from build123d import *

# Parameters (mm, degrees)
SKETCH_1_W      = 53.3
SKETCH_1_H      = 68.6
SKETCH_1_R      = 1.5
EXTRUDE_1_DEPTH = 1.6
SKETCH_2_W      = 11.561255196
SKETCH_2_H      = 12.248286565
SKETCH_2_W_2    = 5.622199285
SKETCH_2_W_3    = 5.780627598
SKETCH_2_H_2    = 42.710987652
SKETCH_2_W_4    = 4.348124609
SKETCH_2_H_3    = 38.380226424
EXTRUDE_2_DEPTH = 10


with BuildPart() as part:
    # 草图1 → 凸台-拉伸1 (new body)
    with BuildSketch(Plane.XY):
        with Locations((-11.140811044, 19.148070952)):
            Rectangle(SKETCH_1_W, SKETCH_1_H)
        with Locations((-19.990811044, 50.948070952)):
            Circle(SKETCH_1_R, mode=Mode.SUBTRACT)
        with Locations((7.909188956, 50.948070952)):
            Circle(SKETCH_1_R, mode=Mode.SUBTRACT)
        with Locations((-32.490811044, 0.148070952)):
            Circle(SKETCH_1_R, mode=Mode.SUBTRACT)
        with Locations((13.009188956, -1.151929048)):
            Circle(SKETCH_1_R, mode=Mode.SUBTRACT)
    extrude(amount=EXTRUDE_1_DEPTH)

    # 草图2 → 凸台-拉伸2 (add)
    with BuildSketch(Plane.XY.offset(1.6)):
        with Locations((-26.811580019, -9.027785766)):
            Rectangle(SKETCH_2_W, SKETCH_2_H)
        with Locations((6.68110059, -9.027785766)):
            Rectangle(SKETCH_2_W_2, SKETCH_2_H)
        with Locations((-29.701893818, 25.423145352)):
            Rectangle(SKETCH_2_W_3, SKETCH_2_H_2)
        with Locations((8.855162896, 27.588525966)):
            Rectangle(SKETCH_2_W_4, SKETCH_2_H_3)
    extrude(amount=EXTRUDE_2_DEPTH)


solid = part.part
Could you check a few things on this model? Use its own coordinates, in mm. A direction names the side the tool comes from. Give positions to 0.01 mm unless a question says otherwise; leave off trailing zeros. Order: outer loops, then holes, each group sorted by start corner. A loop starts at its lowest first (then second) coordinate and runs counter-clockwise, first axis right, second up.
1. Thinking about a two-plate mould opening in X: for faces 5 (the flat face through (-21.031, -9, 7)), 6 (the flat face through (-32.592, 25, 7)), 7 (the flat face through (-27, -9, 11.6)), which applies, +X half, -X half, draft (parallel to the pull), parting line (faces both ways), or undercut?
Answers below:
face 5: undercut
face 6: -X half
face 7: draft
2. Suppose I cut it at D-D (x = -19.5). Write out the boundary of the cut face in (y, z), plus the area to 3 significant figures.
Answers below:
outline: (-15.15, 0) - (49.53, 0) - (49.53, 1.6) - (-15.15, 1.6) - close; (52.37, 0) - (53.45, 0) - (53.45, 1.6) - (52.37, 1.6) - close
area: 105 mm2
3. Suppose I cut it at C-C (y = 31.5). Write out the boundary of the cut face in (x, z).
Answers below:
outline: (-37.79, 0) - (15.51, 0) - (15.51, 1.6) - (11.03, 1.6) - (11.03, 11.6) - (6.68, 11.6) - (6.68, 1.6) - (-26.81, 1.6) - (-26.81, 11.6) - (-32.59, 11.6) - (-32.59, 1.6) - (-37.79, 1.6) - close
4. Suppose I cut it at A-A (z = 8.5). Write out the boundary of the cut face in (x, y).
Answers below:
outline: (-32.59, -15.15) - (-21.03, -15.15) - (-21.03, -2.9) - (-32.59, -2.9) - close; (-32.59, 4.07) - (-26.81, 4.07) - (-26.81, 46.78) - (-32.59, 46.78) - close; (3.87, -15.15) - (9.49, -15.15) - (9.49, -2.9) - (3.87, -2.9) - close; (6.68, 8.4) - (11.03, 8.4) - (11.03, 46.78) - (6.68, 46.78) - close
5. I need wall thicknesses on L1, parallel to X at y = 18, z = 11.25; L2, parallel to X at y = -8, z = 3; L3, parallel to Y at x = -30, z = 3. Which ranges of each line are inside material? Lowest first, please.
Answers below:
L1: x = -32.59 to -26.81, 6.68 to 11.03
L2: x = -32.59 to -21.03, 3.87 to 9.49
L3: y = -15.15 to -2.9, 4.07 to 46.78
6. Which directions (+Z, -Z, +X, -X, +Y, -Y) give clear straight access to the entire face, cutting with the end or side of a thin tool? Please do faces 1 (the flat face through (9.492, -9, 7)), 2 (the flat face through (11.029, 27, 7)), 3 (the flat face through (-32.592, -9, 7)), 4 (the flat face through (9, 8.398, 7)).
Answers below:
face 1: +Z, +X, -Y
face 2: +Z, +X, +Y, -Y
face 3: +Z, -X, +Y, -Y
face 4: +Z, +X
7. Suppose I cut it at B-B (x = -29). Write out the boundary of the cut face in (y, z).
Answers below:
outline: (-15.15, 0) - (53.45, 0) - (53.45, 1.6) - (46.78, 1.6) - (46.78, 11.6) - (4.07, 11.6) - (4.07, 1.6) - (-2.9, 1.6) - (-2.9, 11.6) - (-15.15, 11.6) - close
8. For pin 1 (5 mm diameter, centred on y = -7, z = 6.5, fed in from -X); pin 2 (4.5 mm diameter, centred on x = -30.5, z = 8.5, fed in from +Y); pin 3 (5 mm diameter, centred on y = 18, z = 8.5, fed in from +X), each with a flat end and sliding along its axis, tell me the tip position at first contact or that it passes through.
Answers below:
pin 1: stops at x = -32.59
pin 2: stops at y = 46.78
pin 3: stops at x = 11.03
